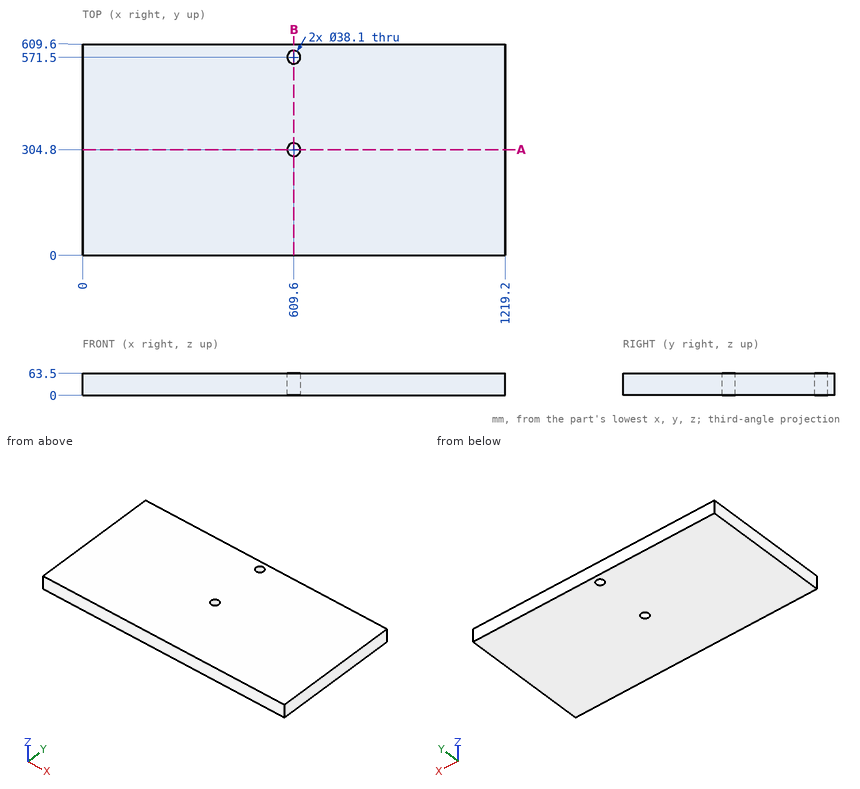
The drawing under review shows one solid part. Ordinate dimensions are in mm from its lowest x, y, z. Round coordinates to 2 decimals unless told otherwise and drop trailing zeros. Loops run counter-clockwise (first coordinate to the right, second up) from the corner with the lowest first, then second, coordinate; pieces in that order, holes last. Notation, with made-up numbers: (62.25, 38.5) - (85.25, 38.5) arc R12 cw to (85.25, 45.5) - close; hole circle Ø7 at (75, 65.25). An arc over 180 degrees is marked (long way). Put each result on its own line as item: value. Start each with the question number.
1. For probe 1 along Y at (x, z) = (609.6, 40.5); probe 2 along X at (y, z) = (571, 28); probe 3 along X at (y, z) = (563, 56), list the stretches that pass through material, from the lowest coordinate up. Write a range as [from, to].
2. Consider section A-A on y = 304.8. State the section outline as (x, z) points.
3. Consider section B-B on x = 609.6. State the section outline as (y, z) points, plus the area to 3 significant figures.
4. Insertion check: P1, Ø23, axis at x = 609.6, y = 571.5, coming from the +Z side. The pin has a flat end and moves straight along its axis. Give the tip position at first contact, or say it passes through.
Result sheet:
1. probe 1: [0, 285.75], [323.85, 552.45], [590.55, 609.6]
1. probe 2: [0, 590.56], [628.64, 1219.2]
1. probe 3: [0, 592.55], [626.65, 1219.2]
2. outline: (0, 0) - (590.55, 0) - (590.55, 63.5) - (0, 63.5) - close; (628.65, 0) - (1219.2, 0) - (1219.2, 63.5) - (628.65, 63.5) - close
3. outline: (0, 0) - (285.75, 0) - (285.75, 63.5) - (0, 63.5) - close; (323.85, 0) - (552.45, 0) - (552.45, 63.5) - (323.85, 63.5) - close; (590.55, 0) - (609.6, 0) - (609.6, 63.5) - (590.55, 63.5) - close
3. area: 33,900 mm^2
4. P1: through
